Input: part model. Units: mm. Frame: model coordinates. A direction names the side the tool comes from. Round coordinates to 2 decimals unless told otherwise and drop trailing zeros. Write each loop counter-clockwise with the first axis right and the second up, starting at its lowest first coordinate (ties: lowest second). Pieces come first, ordered by that corner, then holes. Notation, with made-up numbers: (55, 22.25) -> (83, 22.25) arc R23 cw to (83, 38.25) -> close; hole circle Ø11 at (18, -2). An arc over 180 degrees is marked (long way). Use CSV: the item, a comma, the result in double quotes.
```python
from build123d import *

# Parameters (mm, degrees)
CYLINDER002_R     = 13
CYLINDER002_DEPTH = 120
CYLINDER001_R     = 16
CYLINDER001_DEPTH = 120
FILLET001_R       = 1
CYLINDER003_R     = 13
CYLINDER003_DEPTH = 120
CYLINDER_R        = 19
CYLINDER_DEPTH    = 60
FILLET_R          = 1


with BuildPart() as obj1:
    # Cylinder002 → Cylinder002 (new body)
    with BuildSketch(Plane.XY.offset(-60)):
        Circle(CYLINDER002_R)
    extrude(amount=CYLINDER002_DEPTH)


with BuildPart() as fillet001:
    # Cylinder001 → Cylinder001 (new body)
    with BuildSketch(Plane.XY.offset(-60)):
        Circle(CYLINDER001_R)
    extrude(amount=CYLINDER001_DEPTH)

    # Cut: cut obj1
    add(obj1.part, mode=Mode.SUBTRACT)

    # Fillet001
    fillet001_edges = [fillet001.edges().sort_by_distance(p)[0] for p in [
        (-16, 0, 60),
        (-16, 0, -60),
    ]]
    fillet(fillet001_edges, radius=FILLET001_R)


with BuildPart() as obj2:
    # Cylinder003 → Cylinder003 (new body)
    with BuildSketch(Plane.XY.offset(-60)):
        Circle(CYLINDER003_R)
    extrude(amount=CYLINDER003_DEPTH)


with BuildPart() as fusion:
    # Cylinder → Cylinder (new body)
    with BuildSketch(Plane.XY.offset(-30)):
        Circle(CYLINDER_R)
    extrude(amount=CYLINDER_DEPTH)

    # Cut001: cut obj2
    add(obj2.part, mode=Mode.SUBTRACT)

    # Fillet
    fillet_edges = [fusion.edges().sort_by_distance(p)[0] for p in [
        (-19, 0, 30),
        (-19, 0, -30),
    ]]
    fillet(fillet_edges, radius=FILLET_R)

    # Fusion: union Fillet001
    add(fillet001.part)


solid = fusion.part
```
Item 1: Set-up query: faces 4 (the face through (-3.47, -15.62, -44.7)), 5 (the face through (-0.1, 13.4, -60)), 6 (the face through (-3.47, -15.62, 44.3)). Return all of +Z, -Z, +X, -X, +Y, -Y with unobstructed straight access to the full face (end or side cutting, diameter ignored); none if empty.
Worked answers:
face 4,"-Z"
face 5,"-Z, +X, -X, +Y, -Y"
face 6,"+Z"
Item 2: Line query: line 1 (Y direction, x = 0, z = -1.5); line 2 (Y direction, x = 0, z = 34); line 3 (Z direction, x = -17, y = 6). Output: solid intervals per line, ascending.
Worked answers:
line 1,"y = -19 to -13, 13 to 19"
line 2,"y = -16 to -13, 13 to 16"
line 3,"z = -30 to 30"
Item 3: Section query D-D on z = 18. Return the cut outline in (x, y), plus the area to 3 significant figures.
Worked answers:
outline,"circle Ø38 at (0, 0); hole circle Ø26 at (0, 0)"
area,"603 mm²"
Item 4: First-contact query: pin 1 Ø10 at (x, z) = (3.5, -13.5) entering from -Y; pin 2 Ø1.5 at (x, z) = (-3.5, -7.5) entering from +Y; pin 3 Ø4 at (x, z) = (2.5, -38.5) entering from -Y. Flat tips, straight axial feed; report the tip coordinate or a pass-through.
Worked answers:
pin 1,"stops at y = -19"
pin 2,"stops at y = 18.8"
pin 3,"stops at y = -15.99"
Item 5: Pull-direction query (X, two-part tool) for faces 1 (the face through (8.767, -16.856, -0.406)), 2 (the face through (-10.316, -7.91, -0.84)), 3 (the face through (-0.1, 13.4, 60)); classes: +X half, -X half, draft (parallel to the pull), parting line (faces both ways), or undercut.
Worked answers:
face 1,"parting line"
face 2,"undercut"
face 3,"draft"
Item 6: Section query C-C on z = 40. Return the cut outline in (x, y).
Worked answers:
outline,"circle Ø32 at (0, 0); hole circle Ø26 at (0, 0)"
Item 7: Section query A-A on y = 0. Return the cut outline in (x, z).
Worked answers:
outline,"(-19, -29) arc R1 ccw to (-18, -30) -> (-16, -30) -> (-16, -59) arc R1 ccw to (-15, -60) -> (-13, -60) -> (-13, 60) -> (-15, 60) arc R1 ccw to (-16, 59) -> (-16, 30) -> (-18, 30) arc R1 ccw to (-19, 29) -> close; (13, -60) -> (15, -60) arc R1 ccw to (16, -59) -> (16, -30) -> (18, -30) arc R1 ccw to (19, -29) -> (19, 29) arc R1 ccw to (18, 30) -> (16, 30) -> (16, 59) arc R1 ccw to (15, 60) -> (13, 60) -> close"
